Source: CAD feature listing. Evaluate the final solid. Frame: model axes, mm. Face numbers are marked on the shaded views. A direction names the side the tool comes from. Round coordinates to 2 decimals unless told otherwise and drop trailing zeros. Order: outer loops, then holes, each group sorted by start corner. A loop starts at its lowest first (then second) coordinate and runs counter-clockwise, first axis right, second up. Notation, with made-up numbers: (74, -17) -> (90, -17) arc R13 cw to (90, 5) -> close; hole circle Ø11 at (16.5, -19). An arc over 180 degrees is marked (long way). Answer as CSV lines item,"result".
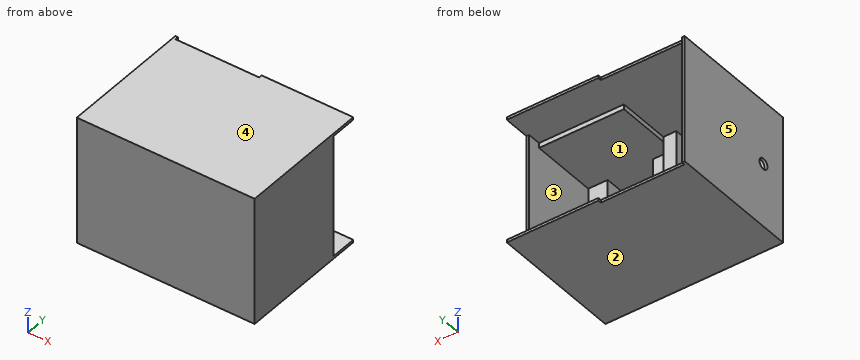
Autodesk Inventor part; units mm, degrees
ref_plane "YZ Plane" through (0, 0, 0) normal (1, 0, 0) x (0, 1, 0)
ref_plane "XZ Plane" through (0, 0, 0) normal (0, 1, 0) x (-1, 0, 0)
ref_plane "XY Plane" through (0, 0, 0) normal (0, 0, 1) x (1, 0, 0)
sketch "Sketch1" plane through (0, 0, 0) normal (0, 1, 0) x (-1, 0, 0)
  line L0 (0, 0) -> (-134, 0)
  line L1 (-134, 0) -> (-134, -96)
  line L2 (-134, -96) -> (0, -96)
  line L3 (0, -96) -> (0, 0)
  line L4 (0, 0) -> (-2, 0)
  line L5 (-2, 0) -> (-2, -2)
  line L6 (-2, -2) -> (0, -2)
  line L7 (0, -2) -> (0, 0)
  line L8 (-134, -96) -> (-132, -96)
  line L9 (-132, -96) -> (-132, -94)
  line L10 (-132, -94) -> (-134, -94)
  line L11 (-134, -94) -> (-134, -96)
  line L12 (-2, -2) -> (-132, -2)
  line L13 (-132, -2) -> (-132, -94)
  line L14 (-132, -94) -> (-2, -94)
  line L15 (-2, -94) -> (-2, -2)
  line L16 (-132, -94) -> (-68, -94)
  line L17 (-68, -94) -> (-68, -74)
  line L18 (-68, -74) -> (-132, -74)
  line L19 (-132, -74) -> (-132, -94)
  line L20 (-132, -2) -> (-68, -2)
  line L21 (-68, -2) -> (-68, -22)
  line L22 (-68, -22) -> (-132, -22)
  line L23 (-132, -22) -> (-132, -2)
  line L24 (-132, -74) -> (-71.6783, -74)
  line L25 (-71.6783, -22) -> (-132, -22)
  line L26 (-71.6783, -74) -> (-71.6783, -22)
  line L27 (-71.6783, -88.5049) -> (-132, -88.5049)
  line L28 (-132, -88.5049) -> (-132, -7.5049)
  line L29 (-132, -7.5049) -> (-71.6783, -7.5049)
  line L30 (-71.6783, -7.5049) -> (-71.6783, -88.5049)
  line L31 (-68, -94) -> (-58.2781, -94)
  line L32 (-58.2781, -94) -> (-58.2781, -2)
  line L33 (-58.2781, -2) -> (-68, -2)
  line L34 (-68, -2) -> (-68, -94)
  line L35 (-2, -94) -> (-58.2781, -94)
  line L36 (-58.2781, -94) -> (-58.2781, -2)
  line L37 (-58.2781, -2) -> (-2, -2)
  line L38 (-2, -2) -> (-2, -94)
  line L39 (-68, -74) -> (-83.3567, -74)
  line L40 (-83.3567, -74) -> (-83.3567, -94)
  line L41 (-83.3567, -94) -> (-68, -94)
  line L42 (-68, -94) -> (-68, -74)
  line L43 (-132, -74) -> (-117.3588, -74)
  line L44 (-117.3588, -74) -> (-117.3588, -94)
  line L45 (-117.3588, -94) -> (-132, -94)
  line L46 (-132, -94) -> (-132, -74)
  line L47 (-68, -22) -> (-83.3567, -22)
  line L48 (-83.3567, -22) -> (-83.3567, -2)
  line L49 (-83.3567, -2) -> (-68, -2)
  line L50 (-68, -2) -> (-68, -22)
  line L51 (-117.3588, -22) -> (-132, -22)
  line L52 (-132, -22) -> (-132, -2)
  line L53 (-132, -2) -> (-117.3588, -2)
  line L54 (-117.3588, -2) -> (-117.3588, -22)
  line L55 (-68, -5.7143) -> (-132, -5.7143)
  line L56 (-132, -5.7143) -> (-132, -2)
  line L57 (-132, -2) -> (-68, -2)
  line L58 (-68, -2) -> (-68, -5.7143)
  line L59 (-68, -94) -> (-132, -94)
  line L60 (-132, -94) -> (-132, -90.4872)
  line L61 (-132, -90.4872) -> (-68, -90.4872)
  line L62 (-68, -90.4872) -> (-68, -94)
  line L63 (-132, -92.2436) -> (-29, -92.2436)
  line L64 (-29, -92.2436) -> (-29, -2.2436)
  line L65 (-29, -2.2436) -> (-132, -2.2436)
  line L66 (-132, -2.2436) -> (-132, -92.2436)
  point P0 (-83.3567, -2)
  point P1 (-83.3567, -7.5049)
  point P2 (-117.3588, -7.5049)
  point P3 (-132, -7.5049)
  point P4 (-132, -88.5049)
  point P5 (-117.3588, -88.5049)
  point P6 (-83.3567, -88.5049)
  dimension "d0" = 134
  dimension "d1" = 96
  dimension "d2" = 2
  dimension "d3" = 2
  dimension "d4" = 2
  dimension "d5" = 2
  dimension "d6" = 64
  dimension "d7" = 64
  dimension "d9" = 20
  dimension "d10" = 20
  dimension "d11" = 81
  dimension "d22" = 5.5049
  dimension "d23" = 90
  dimension "d24" = 103
extrude "Extrusion1" add sketch "Sketch1" along normal blind 100 contours L3 L6 L5 L0 | L5 L12 L13 L10 L1 L0 | L3 L2 L9 L14 L15 L6 | L10 L9 L2 L1
extrude "Extrusion2" add sketch "Sketch1" along normal blind 20 contours L13 L63 L44 L14 | L21 L65 L48 L12 | L13 L61 L44 L63 | L21 L55 L48 L65 | L14 L40 L63 L17 | L13 L27 L44 L61 | L54 L65 L13 L12 | L21 L22 L30 L29 L48 L55 | L63 L40 L61 L17 | L13 L18 L44 L27 | L54 L55 L13 L65 | L61 L40 L27 L30 L18 L17 | L54 L29 L13 L55 | L29 L30 L22 L48 | L13 L29 L54 L22 | L40 L18 L30 L27
extrude "Extrusion3" add sketch "Sketch1" along normal blind 30 contours L32 L65 L21 L12 | L32 L63 L17 L34 L21 L65 | L14 L17 L63 L32
extrude "Extrusion4" add sketch "Sketch1" along normal blind 2 contours L15 L14 L32 L63 L64 L65 L12 | L65 L64 L63 L32 | L44 L63 L40 L14 | L48 L65 L54 L12 | L44 L61 L40 L63 | L48 L55 L54 L65 | L13 L18 L44 L27 | L44 L27 L40 L61 | L48 L29 L54 L55 | L34 L18 L26 L22 | L13 L22 L26 L18 | L44 L18 L40 L27 | L48 L22 L54 L29 | L29 L30 L22 L48 | L13 L29 L54 L22 | L40 L18 L30 L27
sketch "Sketch2" plane through (0, 0, 0) normal (0, 0, 1) x (1, 0, 0)
  line L0 (132, 20) -> (132, 100)
  line L1 (132, 70) -> (60, 70)
  line L2 (83.3567, 20) -> (68, 20)
  line L3 (60, 70) -> (132, 70)
  line L4 (132, 70) -> (132, 65.2658)
  line L5 (132, 65.2658) -> (60, 65.2658)
  line L6 (60, 65.2658) -> (60, 70)
  point P0 (0, 0)
  dimension "d20" = 50
  dimension "d21" = 72
extrude "Extrusion5" add sketch "Sketch1" along normal blind 70 contours L13 L63 L44 L14 | L21 L65 L48 L12 | L13 L61 L44 L63 | L44 L63 L40 L14 | L48 L65 L54 L12 | L21 L55 L48 L65 | L14 L40 L63 L17 | L44 L61 L40 L63 | L54 L65 L13 L12 | L48 L55 L54 L65 | L63 L40 L61 L17 | L54 L55 L13 L65
sketch "Sketch3" plane through (0, 100, 0) normal (0, 1, 0) x (1, 0, 0)
  line L0 (0, 0) -> (134, 0)
  line L1 (2.0076, 96.0653) -> (65.0076, 96.0653)
  line L2 (65.0076, 96.0653) -> (65.0076, 0)
  line L3 (65.0076, 0) -> (2.0076, 0)
  line L4 (2.0076, 0) -> (2.0076, 96.0653)
  dimension "d27" = 63
extrude "Extrusion6" cut sketch "Sketch3" against normal blind 2.5
sketch "Sketch4" plane through (0, 0, -96) normal (-1, 0, 0) x (0, 0, 1)
  line L0 (2, 2) -> (2, 100)
  line L1 (94, 2) -> (2, 2)
  line L2 (2, 2) -> (94, 2)
  circle A0 centre (48, 20.0516) radius 4
  point P0 (96, 0)
  dimension "d30" = 8
sketch "Sketch5" plane through (0, 100, 0) normal (0, 1, 0) x (1, 0, 0)
  line L0 (134, 0) -> (134, 96)
  line L1 (132, 94) -> (134, 94)
  line L2 (134, 94) -> (134, 2)
  line L3 (134, 2) -> (132, 2)
  line L4 (132, 2) -> (132, 94)
  point P0 (0, 0)
  dimension "d31" = 92
extrude "Extrusion7" cut sketch "Sketch5" against normal blind 20
extrude "Extrusion8" cut sketch "Sketch4" against normal blind 20
properties part number "FINALE"
1. Reachability of the marked faces 1 and 2 from +Z, -Z, +X, -X, +Y, -Y: full face, straight path, thin tool, end or side. Return the list, or none.
Results below:
face 1,"+Y"
face 2,"-Z, +X, -X, +Y, -Y"
2. Pin query (flat end, axial travel): pin 1 (2 mm diameter, centred on x = 133, z = -64.5, fed in from +Y); pin 2 (2 mm diameter, centred on x = 41.5, z = -94.5, fed in from +Y); pin 3 (5 mm diameter, centred on x = 62.5, z = -64.5, fed in from +Y). Return the tip coordinate at first contact, or that it passes through.
Results below:
pin 1,"y = 80"
pin 2,"y = 97.5"
pin 3,"y = 30"
3. Line query: L1, parallel to X at y = 4.5, z = -82.5; L2, parallel to X at y = 11.5, z = -42; L3, parallel to Z at x = 47, y = 54. Output: solid intervals per line, ascending. Write a range as [from, to].
Results below:
L1,"[0, 2], [58.28, 83.36], [117.36, 134]"
L2,"[0, 2], [58.28, 68], [132, 134]"
L3,"[-96, -94], [-2, 0]"
4. Section query A-A on y = 6. Return loops of the section in (x, z).
Results below:
outline,"(0, -96) -> (134, -96) -> (134, 0) -> (0, 0) -> close; hole (2, -94) -> (58.28, -94) -> (58.28, -2) -> (2, -2) -> close; hole (68, -74) -> (83.36, -74) -> (83.36, -90.49) -> (117.36, -90.49) -> (117.36, -74) -> (132, -74) -> (132, -22) -> (117.36, -22) -> (117.36, -5.71) -> (83.36, -5.71) -> (83.36, -22) -> (68, -22) -> close"
5. Section query C-C on y = 87. Return loops of the section in (x, z), and give its area (3 significant figures).
Results below:
outline,"(0, -96) -> (134, -96) -> (134, -94) -> (2, -94) -> (2, -2) -> (134, -2) -> (134, 0) -> (0, 0) -> close"
area,"720 mm2"
6. Section query B-B on z = -48. Return loops of the section in (x, y).
Results below:
outline,"(0, 0) -> (134, 0) -> (134, 80) -> (132, 80) -> (132, 2) -> (68, 2) -> (68, 30) -> (58.28, 30) -> (58.28, 2) -> (2, 2) -> (2, 16.05) -> (0, 16.05) -> close; (0, 24.05) -> (2, 24.05) -> (2, 100) -> (0, 100) -> close"
7. Mould query, pull axis Z, two halves, no side actions, for the marked faces 3, 4 and 5. Classes: released by +Z, released by -Z, zero draft, split by the parting line, or undercut.
Results below:
face 3,"undercut"
face 4,"released by +Z"
face 5,"zero draft"
8. Section query D-D on x = 41.5. Return loops of the section in (y, z).
Results below:
outline,"(0, -96) -> (97.5, -96) -> (97.5, -94) -> (2, -94) -> (2, -2) -> (97.5, -2) -> (97.5, 0) -> (0, 0) -> close"
